Here's how the part is built. I have some questions about the finished solid (model axes, mm). A direction names the side the tool comes from. Coordinates: 2 decimals unless noted, no trailing zeros. Order: outer loops, then holes, each group sorted by start corner. A loop starts at its lowest first (then second) coordinate and runs counter-clockwise, first axis right, second up. Notation, with made-up numbers: (63, -30) - (94, -30) arc R25 ccw to (94, 9) - close; hole circle Ø1 at (24, 3.5). An arc over 180 degrees is marked (long way). Answer as CSV lines item,"result". Start each with the question number.
Q1. For faces 1 (the face through (-30, 22, -30)), 2 (the face through (16, 9, 0)), 3 (the face through (-30, 22, 30)), 4 (the face through (12.4, -34.1, 6.5)), 5 (the face through (5.5, -42, -5.5)), which set-ups out of +Z, -Z, +X, -X, +Y, -Y let a thin tool reach every point of the face, with its end or its side?
Q2. I need wall thicknesses on line 1 (Y direction, x = -22.5, z = 31.05); line 2 (Z direction, x = -16, y = -15); line 3 (X direction, y = -7.5, z = 18.5). Which ranges of each line are inside material? Lowest first, please.
Q3. Suppose I cut it at D-D (z = 9.5). Please give me the cut outline in (x, y).
Q4. For pin 1 Ø8 at (x, y) = (-18.5, -13) entering from -Z; pin 2 Ø2.5 at (x, y) = (-22.5, 22.5) entering from -Z; pin 3 Ø2 at (x, z) = (-29.5, 27.5) entering from +Y; pin 4 Ø4 at (y, z) = (-6, 25.5) entering from -X, each with a flat end and sliding along its axis, tell me the tip position at first contact or that it passes through.
Q5. Suppose I cut it at C-C (x = 0). Please give me the cut outline in (y, z).
Q6. Suppose I cut it at B-B (z = 18). Please give me the cut outline in (x, y), then the cut area to 3 significant figures.
Q7. Suppose I cut it at A-A (y = 5.5). Please give me the cut outline in (x, z), then the cut area to 3 significant figures.
Q8. Thinking about a two-plate mould opening in Y: for faces 6 (the face through (-23.61, 23.01, 31.48)), 7 (the face through (-30, 12, 30)), 8 (the face through (-29.49, 27.15, -0.42)), which applies, released by +Y, released by -Y, zero draft, split by the parting line, or undercut?
from build123d import *

# Parameters (mm, degrees)
SALIENTE_EXTRUIR1_DEPTH = 30
CROQUIS2_R              = 4
CROQUIS2_R_2            = 1.5
CROQUIS2_W              = 2.6
CROQUIS2_H              = 10
SALIENTE_EXTRUIR2_DEPTH = 3
REDONDEO1_R             = 10
REDONDEO2_R             = 5
CORTAR_EXTRUIR1_DEPTH   = 50


with BuildPart() as part:
    # Croquis1 → Saliente-Extruir1 (new, symmetric)
    with BuildSketch(Plane.XY):
        with BuildLine():
            Line((-32.5, 30), (-16, 30))
            Line((-16, 30), (-16, 0))
            ThreePointArc((-16, 0), (0, -16), (16, 0))
            Line((16, 0), (16, 30))
            Line((16, 30), (32.5, 30))
            Line((32.5, 30), (32.5, -30))
            Line((32.5, -30), (-32.5, -30))
            Line((-32.5, -30), (-32.5, 30))
        make_face()
    extrude(amount=SALIENTE_EXTRUIR1_DEPTH, both=True)

    # Croquis2 → Saliente-Extruir2 (add)
    # profile 1 of 2: a face of its own
    with BuildSketch(Plane.XY.offset(30)):
        with Locations((-22.5, 22)):
            Circle(CROQUIS2_R)
        with Locations((-22.5, 22)):
            Circle(CROQUIS2_R_2, mode=Mode.SUBTRACT)
    # profile 2 of 2: a face of its own
    with BuildSketch(Plane.XY.offset(30)):
        with Locations((-29.7, 17)):
            Rectangle(CROQUIS2_W, CROQUIS2_H)
    saliente_extruir2 = extrude(amount=SALIENTE_EXTRUIR2_DEPTH)

    # Croquis4 → Revolución1 (revolve)
    with BuildSketch(Plane.XY, mode=Mode.PRIVATE) as revoluci_n1_sk:
        Polygon((0, -30), (14, -30), (14, -38), (7.3, -38), (7.3, -42), (12.7, -42), (12.7, -46), (0, -46), align=None)
    revolve(revoluci_n1_sk.sketch.rotate(Axis((0, -19.505365955, 0), (0, -1, 0)), 90), axis=Axis((0, -19.505365955, 0), (0, -1, 0)))

    # Simetría2: Saliente-Extruir2 across plane
    add(saliente_extruir2.mirror(Plane.XY))

    # Redondeo1
    # the kernel refuses this fillet: 10 mm, written as the material it takes off along each edge
    with BuildSketch(Plane(origin=(32.5, 55, -30), x_dir=(-1, 0, 0), z_dir=(0, -1, 0)), Plane(origin=(-32.5, 30, -55), x_dir=(1, 0, 0), z_dir=(0, 0, 1)), Plane(origin=(32.5, -30, -55), x_dir=(-1, 0, 0), z_dir=(0, 0, 1)), Plane(origin=(-32.5, -30, -55), x_dir=(0, 1, 0), z_dir=(0, 0, 1))) as redondeo1_piece_1:
        with BuildLine():
            CenterArc((REDONDEO1_R, -REDONDEO1_R), REDONDEO1_R, 90, 90)
            Line((0, -REDONDEO1_R), (0, 0))
            Line((0, 0), (REDONDEO1_R, 0))
        make_face()
    extrude(amount=110, mode=Mode.SUBTRACT)
    with BuildSketch(Plane(origin=(-32.5, -55, -30), x_dir=(0, 0, 1), z_dir=(0, 1, 0))) as redondeo1_piece_2_section:
        with BuildLine():
            CenterArc((REDONDEO1_R, REDONDEO1_R), REDONDEO1_R, 180, 90)
            Line((0, REDONDEO1_R), (0, 0))
            Line((0, 0), (REDONDEO1_R, 0))
        make_face()
    redondeo1_piece_2 = extrude(amount=110, mode=Mode.PRIVATE)
    redondeo1_piece_2 = split(redondeo1_piece_2, bisect_by=Plane(origin=(-31, -9, -26.666087893), z_dir=(-1, 0, 0)), keep=Keep.TOP, mode=Mode.PRIVATE)
    add(redondeo1_piece_2, mode=Mode.SUBTRACT)
    with BuildSketch(Plane(origin=(-32.5, -55, -30), x_dir=(0, 0, 1), z_dir=(0, 1, 0))) as redondeo1_piece_3_section:
        with BuildLine():
            CenterArc((REDONDEO1_R, REDONDEO1_R), REDONDEO1_R, 180, 90)
            Line((0, REDONDEO1_R), (0, 0))
            Line((0, 0), (REDONDEO1_R, 0))
        make_face()
    redondeo1_piece_3 = extrude(amount=110, mode=Mode.PRIVATE)
    redondeo1_piece_3 = split(redondeo1_piece_3, bisect_by=Plane(origin=(-29.890039843, 12, -28.324282077), z_dir=(0, -1, 0)), keep=Keep.TOP, mode=Mode.PRIVATE)
    add(redondeo1_piece_3, mode=Mode.SUBTRACT)
    with BuildSketch(Plane(origin=(-32.5, -55, -30), x_dir=(0, 0, 1), z_dir=(0, 1, 0))) as redondeo1_piece_4_section:
        with BuildLine():
            CenterArc((REDONDEO1_R, REDONDEO1_R), REDONDEO1_R, 180, 90)
            Line((0, REDONDEO1_R), (0, 0))
            Line((0, 0), (REDONDEO1_R, 0))
        make_face()
    redondeo1_piece_4 = extrude(amount=110, mode=Mode.PRIVATE)
    redondeo1_piece_4 = split(redondeo1_piece_4, bisect_by=Plane(origin=(-28.4, 16.722523597, -29.405754559), z_dir=(1, 0, 0)), keep=Keep.TOP, mode=Mode.PRIVATE)
    redondeo1_piece_4 = redondeo1_piece_4 - Plane(origin=(-22.5, 22, -29.405754559), x_dir=(1, 0, 0), z_dir=(0, 0, 1)) * Cylinder(4, 260, mode=Mode.PRIVATE)
    add(redondeo1_piece_4, mode=Mode.SUBTRACT)
    with BuildSketch(Plane(origin=(-32.5, -55, -30), x_dir=(0, 0, 1), z_dir=(0, 1, 0))) as redondeo1_piece_5_section:
        with BuildLine():
            CenterArc((REDONDEO1_R, REDONDEO1_R), REDONDEO1_R, 180, 90)
            Line((0, REDONDEO1_R), (0, 0))
            Line((0, 0), (REDONDEO1_R, 0))
        make_face()
    redondeo1_piece_5 = extrude(amount=110, mode=Mode.PRIVATE)
    redondeo1_piece_5 = split(redondeo1_piece_5, bisect_by=Plane(origin=(-29.890039843, 22, -28.324282077), z_dir=(0, 1, 0)), keep=Keep.TOP, mode=Mode.PRIVATE)
    redondeo1_piece_5 = split(redondeo1_piece_5, bisect_by=Plane(origin=(-28.4, 26, -28.324282077), z_dir=(-1, 0, 0)), keep=Keep.TOP, mode=Mode.PRIVATE)
    add(redondeo1_piece_5, mode=Mode.SUBTRACT)
    with BuildSketch(Plane(origin=(32.5, 55, 30), x_dir=(-1, 0, 0), z_dir=(0, -1, 0)), Plane(origin=(32.5, 30, 55), x_dir=(0, -1, 0), z_dir=(0, 0, -1))) as redondeo1_piece_6:
        with BuildLine():
            CenterArc((REDONDEO1_R, REDONDEO1_R), REDONDEO1_R, 180, 90)
            Line((0, REDONDEO1_R), (0, 0))
            Line((0, 0), (REDONDEO1_R, 0))
        make_face()
    extrude(amount=110, mode=Mode.SUBTRACT)
    with BuildSketch(Plane(origin=(-32.5, -55, 30), x_dir=(0, 0, -1), z_dir=(0, 1, 0))) as redondeo1_piece_7_section:
        with BuildLine():
            CenterArc((REDONDEO1_R, -REDONDEO1_R), REDONDEO1_R, 90, 90)
            Line((0, -REDONDEO1_R), (0, 0))
            Line((0, 0), (REDONDEO1_R, 0))
        make_face()
    redondeo1_piece_7 = extrude(amount=110, mode=Mode.PRIVATE)
    redondeo1_piece_7 = split(redondeo1_piece_7, bisect_by=Plane(origin=(-31, -9, 26.666087893), z_dir=(-1, 0, 0)), keep=Keep.TOP, mode=Mode.PRIVATE)
    add(redondeo1_piece_7, mode=Mode.SUBTRACT)
    with BuildSketch(Plane(origin=(-32.5, -55, 30), x_dir=(0, 0, -1), z_dir=(0, 1, 0))) as redondeo1_piece_8_section:
        with BuildLine():
            CenterArc((REDONDEO1_R, -REDONDEO1_R), REDONDEO1_R, 90, 90)
            Line((0, -REDONDEO1_R), (0, 0))
            Line((0, 0), (REDONDEO1_R, 0))
        make_face()
    redondeo1_piece_8 = extrude(amount=110, mode=Mode.PRIVATE)
    redondeo1_piece_8 = split(redondeo1_piece_8, bisect_by=Plane(origin=(-29.890039843, 12, 28.324282077), z_dir=(0, -1, 0)), keep=Keep.TOP, mode=Mode.PRIVATE)
    add(redondeo1_piece_8, mode=Mode.SUBTRACT)
    with BuildSketch(Plane(origin=(-32.5, -55, 30), x_dir=(0, 0, -1), z_dir=(0, 1, 0))) as redondeo1_piece_9_section:
        with BuildLine():
            CenterArc((REDONDEO1_R, -REDONDEO1_R), REDONDEO1_R, 90, 90)
            Line((0, -REDONDEO1_R), (0, 0))
            Line((0, 0), (REDONDEO1_R, 0))
        make_face()
    redondeo1_piece_9 = extrude(amount=110, mode=Mode.PRIVATE)
    redondeo1_piece_9 = split(redondeo1_piece_9, bisect_by=Plane(origin=(-28.4, 16.722523597, 29.405754559), z_dir=(1, 0, 0)), keep=Keep.TOP, mode=Mode.PRIVATE)
    redondeo1_piece_9 = redondeo1_piece_9 - Plane(origin=(-22.5, 22, 29.405754559), x_dir=(1, 0, 0), z_dir=(0, 0, -1)) * Cylinder(4, 260, mode=Mode.PRIVATE)
    add(redondeo1_piece_9, mode=Mode.SUBTRACT)
    with BuildSketch(Plane(origin=(-32.5, -55, 30), x_dir=(0, 0, -1), z_dir=(0, 1, 0))) as redondeo1_piece_10_section:
        with BuildLine():
            CenterArc((REDONDEO1_R, -REDONDEO1_R), REDONDEO1_R, 90, 90)
            Line((0, -REDONDEO1_R), (0, 0))
            Line((0, 0), (REDONDEO1_R, 0))
        make_face()
    redondeo1_piece_10 = extrude(amount=110, mode=Mode.PRIVATE)
    redondeo1_piece_10 = split(redondeo1_piece_10, bisect_by=Plane(origin=(-29.890039843, 22, 28.324282077), z_dir=(0, 1, 0)), keep=Keep.TOP, mode=Mode.PRIVATE)
    redondeo1_piece_10 = split(redondeo1_piece_10, bisect_by=Plane(origin=(-28.4, 26, 28.324282077), z_dir=(-1, 0, 0)), keep=Keep.TOP, mode=Mode.PRIVATE)
    add(redondeo1_piece_10, mode=Mode.SUBTRACT)

    # Redondeo2
    redondeo2_edges = [part.edges().sort_by_distance(p)[0] for p in [
        (-16, 30, 0),
        (16, 30, 0),
    ]]
    fillet(redondeo2_edges, radius=REDONDEO2_R)

    # Croquis5 → Cortar-Extruir1 (cut, symmetric)
    with BuildSketch(Plane.XY):
        with BuildLine():
            ThreePointArc((16, 18.087120501), (24.958618735, 19.745432896), (32.5, 14.633249581))
            Line((32.5, 14.633249581), (32.5, 20))
            ThreePointArc((32.5, 20), (29.571067812, 27.071067812), (22.5, 30))
            Line((22.5, 30), (21, 30))
            ThreePointArc((21, 30), (17.464466094, 28.535533906), (16, 25))
            Line((16, 25), (16, 18.087120501))
        make_face()
    extrude(amount=CORTAR_EXTRUIR1_DEPTH, both=True, mode=Mode.SUBTRACT)


solid = part.part
Here are the results:
1,face 1,"-Z, -X, +Y"
1,face 2,"+Z, -Z, +Y"
1,face 3,"+Z, -X, +Y"
1,face 4,"-Y"
1,face 5,"none"
2,line 1,"y = 18 to 20.5, 23.5 to 26"
2,line 2,"z = -30 to 30"
2,line 3,"x = -32.5 to -14.13, 14.13 to 32.5"
3,outline,"(-32.5, -20) arc R10 ccw to (-22.5, -30) - (-10.28, -30) - (-10.28, -38) - (10.28, -38) - (10.28, -30) - (22.5, -30) arc R10 ccw to (32.5, -20) - (32.5, 14.63) arc R12 ccw to (16, 18.09) - (16, 0) arc R16 cw to (-16, 0) - (-16, 25) arc R5 ccw to (-21, 30) - (-22.5, 30) arc R10 ccw to (-32.5, 20) - close; (-8.43, -46) - (8.43, -46) - (8.43, -42) - (-8.43, -42) - close"
4,pin 1,"stops at z = -30"
4,pin 2,"stops at z = -33"
4,pin 3,"stops at y = 28"
4,pin 4,"stops at x = -31.87"
5,outline,"(-46, -12.7) - (-42, -12.7) - (-42, -7.3) - (-38, -7.3) - (-38, -14) - (-30, -14) - (-30, -30) - (-16, -30) - (-16, 30) - (-30, 30) - (-30, 14) - (-38, 14) - (-38, 7.3) - (-42, 7.3) - (-42, 12.7) - (-46, 12.7) - close"
6,outline,"(-32.5, -20) arc R10 ccw to (-22.5, -30) - (22.5, -30) arc R10 ccw to (32.5, -20) - (32.5, 14.63) arc R12 ccw to (16, 18.09) - (16, 0) arc R16 cw to (-16, 0) - (-16, 25) arc R5 ccw to (-21, 30) - (-22.5, 30) arc R10 ccw to (-32.5, 20) - close"
6,area,"2,280 mm²"
7,outline,"(-32.5, -20) arc R10 ccw to (-22.5, -30) - (-16, -30) - (-16, 30) - (-22.5, 30) arc R10 ccw to (-32.5, 20) - close; (16, -30) - (22.5, -30) arc R10 ccw to (32.5, -20) - (32.5, 20) arc R10 ccw to (22.5, 30) - (16, 30) - close"
7,area,"1,890 mm²"
8,face 6,"undercut"
8,face 7,"released by -Y"
8,face 8,"released by +Y"
